Read the model definition and answer for the solid it produces. Units are mm, in the model's axes. A direction names the side the tool comes from. Give positions to 0.01 mm unless a question says otherwise; leave off trailing zeros. Order: outer loops, then holes, each group sorted by start corner. A loop starts at its lowest first (then second) coordinate and runs counter-clockwise, first axis right, second up. Notation, with made-up numbers: (-39, 70.5) - (-24, 70.5) arc R26 ccw to (-24, 101.5) - close; hole circle Ø6 at (86.25, 29.25). An arc over 180 degrees is marked (long way). Return JSON: item names as keys, results as strings.
```python
from build123d import *

# Parameters (mm, degrees)
SKETCH1_R           = 1.45
BOSS_EXTRUDE1_DEPTH = 10
SKETCH2_R           = 2.75
BOSS_EXTRUDE2_DEPTH = 1.6
FILLET1_R           = 1


with BuildPart() as part:
    # Sketch1 → Boss-Extrude1 (new body)
    with BuildSketch(Plane(origin=(0, 0, 0), x_dir=(1, 0, 0), z_dir=(0, 1, 0))):
        with Locations(Location((0, 0, 0), (0, 0, 270))):
            Circle(SKETCH1_R)
    extrude(amount=-BOSS_EXTRUDE1_DEPTH)

    # Sketch2 → Boss-Extrude2 (add)
    with BuildSketch(Plane(origin=(0, 0, 0), x_dir=(1, 0, 0), z_dir=(0, 1, 0))):
        with Locations(Location((0, 0, 0), (0, 0, 270))):
            Circle(SKETCH2_R)
    extrude(amount=BOSS_EXTRUDE2_DEPTH)

    # Fillet1
    fillet1_edges = [part.edges().sort_by_distance(p)[0] for p in [
        (0, 1.6, -2.75),
    ]]
    fillet(fillet1_edges, radius=FILLET1_R)


solid = part.part
```
Q1. A cutting plane is placed at C-C (y = -4). Write down the section's boundary in (x, z), and give its area (3 significant figures).
Values:
{"outline": "circle Ø2.9 at (0, 0)", "area": "6.61 mm²"}
Q2. A cutting plane is placed at B-B (x = 0). Write down the section's boundary in (y, z).
Values:
{"outline": "(-10, -1.45) - (0, -1.45) - (0, -2.75) - (0.6, -2.75) arc R1 ccw to (1.6, -1.75) - (1.6, 1.75) arc R1 ccw to (0.6, 2.75) - (0, 2.75) - (0, 1.45) - (-10, 1.45) - close"}
Q3. Consider L1, parallel to Z at x = 0.5, y = -2.25; L2, parallel to Z at x = 0.6, y = -2.75; L3, parallel to Y at x = -1.9, z = -0.15. Determine where each line is inside the solid, lowest interval first.
Values:
{"L1": "z = -1.36 to 1.36", "L2": "z = -1.32 to 1.32", "L3": "y = 0 to 1.59"}
Q4. A cutting plane is placed at A-A (z = 0). Write down the section's boundary in (x, y).
Values:
{"outline": "(-2.75, 0) - (-1.45, 0) - (-1.45, -10) - (1.45, -10) - (1.45, 0) - (2.75, 0) - (2.75, 0.6) arc R1 ccw to (1.75, 1.6) - (-1.75, 1.6) arc R1 ccw to (-2.75, 0.6) - close"}
Q5. For faces 1 (the flat face through (0, 1.6, 0)), 2 (the cylindrical face through (0.06, -4.93, -1.45)), determine the directions among +Z, -Z, +X, -X, +Y, -Y from which every point of the face is accessible in a straight line to the end or side of a thin tool.
Values:
{"face 1": "+Z, -Z, +X, -X, +Y", "face 2": "-Y"}
Q6. Given pin 1 (2 mm diameter, centred on x = -2, z = 1.5, fed in from -Y), flat-ended and moving along its own axis, determine where the tip first touches the part or whether it passes through.
Values:
{"pin 1": "stops at y = 0"}
